Could you check a few things on this model? Use its own coordinates, in mm. A direction names the side the tool comes from. Give positions to 0.01 mm unless a question says otherwise; leave off trailing zeros. Write each loop counter-clockwise with the first axis right and the second up, starting at its lowest first coordinate (ties: lowest second). Pieces come first, ordered by that corner, then holes. Notation, with made-up numbers: (17.25, 28.25) - (42.25, 28.25) arc R24 ccw to (42.25, 65.25) - close; hole circle Ø5 at (89.25, 36). An arc over 180 degrees is marked (long way). Use one line per item in the form item = value.
Autodesk Inventor part; units mm, degrees
ref_plane "YZ Plane" through (0, 0, 0) normal (1, 0, 0) x (0, 1, 0)
ref_plane "XZ Plane" through (0, 0, 0) normal (0, 1, 0) x (-1, 0, 0)
ref_plane "XY Plane" through (0, 0, 0) normal (0, 0, 1) x (1, 0, 0)
sketch "Sketch1" plane through (0, 0, 0) normal (0, 0, 1) x (1, 0, 0)
  circle A0 centre (0, 0) radius 38.1
  dimension "d0" = 76.2
extrude "Extrusion1" add sketch "Sketch1" along normal blind 25.4
fillet "Fillet1" radius 6.35 2 edges at (-38.1, 0, 25.4) (-38.1, 0, 0)
sketch "Sketch3" plane through (0, 0, 25.4) normal (0, 0, 1) x (1, 0, 0)
  line L0 (6.35, 44.45) -> (-53.2838, 44.45)
  circle A0 centre (0, 0) radius 38.1
  arc A1 (-4.3231, -4.6511) -> (6.35, 0) centre (0, 0) ccw
  line L1 (6.35, 0) -> (6.35, 44.45)
  arc A2 (-53.2838, 44.45) -> (-47.6982, 35.6648) centre (-39.6513, 46.9493) ccw
  line L2 (-50.3182, 38.1) -> (-4.3231, -4.6511)
  dimension "d8" = 44.45
  dimension "d9" = 76.2
  dimension "d10" = 12.7
extrude "Extrusion2" add sketch "Sketch3" along normal blind 3.175 contours L1 A0 L2 A2 L0 | L1 A1 L2 A0 picked at (-4.398, 10.0922)
pattern_linear "Rectangular Pattern1" count 2 spacing 28.575 along (0, 0, -1) of "Extrusion2"
sketch "Sketch4" plane through (-53.2838, 44.45, 25.4) normal (0, 1, 0) x (1, 0, 0)
  line L0 (59.6338, -3.175) -> (0, -3.175)
  line L1 (59.6338, 28.575) -> (0, 28.575)
  line L2 (0, -3.175) -> (59.6338, -3.175)
  line L3 (59.6338, -3.175) -> (59.6338, 28.575)
  line L4 (59.6338, 28.575) -> (0, 28.575)
  line L5 (0, 28.575) -> (0, -3.175)
  point P0 (53.2838, 25.4)
  dimension "d20" = 31.75
extrude "Extrusion3" add sketch "Sketch4" along normal blind 3.175
sketch "Sketch5" plane through (-53.2838, 47.625, 25.4) normal (0, 1, 0) x (1, 0, 0)
  circle A0 centre (19.7076, 12.7) radius 25.4
  line L0 (59.6338, 28.575) -> (0, 28.575)
  line L1 (59.6338, -3.175) -> (59.6338, 28.575)
  dimension "d19" = 15.875
  dimension "d21" = 50.8
extrude "Extrusion4" add sketch "Sketch5" along normal blind 3.175
equation "\"d19\" = 0.5 * d20"
properties part number "Caster Placeholder" material "Aluminum 6061"
1. Imagine slicing it at B-B, the plane z = 12.7. List the corners of the cut face in (x, y) for me (3 decimals).
Response values:
outline = (-58.976, 47.625) - (-53.284, 47.625) - (-53.284, 44.45) - (6.35, 44.45) - (6.35, 47.625) - (-8.176, 47.625) - (-8.176, 50.8) - (-58.976, 50.8) - close; circle Ø76.2 at (0, 0)
2. If we mould it in two halves opening along Z, with no side actions, what happens to faces 1 (the face through (-24, 44.45, 13)), 2 (the face through (6.35, 31, 26)), 3 (the face through (7, -7, 0))? For each: pulls with the +Z half, pulls with the -Z half, needs draft (parallel to the pull), parting line crosses it, or undercut.
Response values:
face_1 = undercut
face_2 = needs draft
face_3 = pulls with the -Z half
3. If I drill on line 1 (Z direction, x = -21, y = -8); line 2 (Z direction, x = -37, y = 47.5) (3 decimals); line 3 (Y direction, x = -41, z = 29) (3 decimals), over which ranges is the centre line in solid material (lowest first)? Write a range as from..to.
Response values:
line_1 = 0..25.4
line_2 = -3.175..28.575
line_3 = 47.625..50.8
4. Imagine slicing it at C-C, the plane z = 20.5. List the corners of the cut face in (x, y) for me (3 decimals).
Response values:
outline = (-57.749, 47.625) - (-53.284, 47.625) - (-53.284, 44.45) - (6.35, 44.45) - (6.35, 47.625) - (-9.403, 47.625) - (-9.403, 50.8) - (-57.749, 50.8) - close; circle Ø75.864 at (0, 0)
5. For pin 1 (8.5 mm diameter, centred on x = -14, y = 26.5, fed in from +Z) (3 decimals); pin 2 (12 mm diameter, centred on x = -45.5, y = 29.5, fed in from -Z) (3 decimals); pin 3 (22.5 mm diameter, centred on x = -37, z = 24.5, fed in from -Y), each with a flat end and sliding along its axis, tell me the tip position at first contact or that it passes through.
Response values:
pin_1 = 28.575
pin_2 = -3.175
pin_3 = -27.16
6. Imagine slicing it at A-A, the plane x = 0. List the corners of the cut face in (y, z) for me (3 decimals), and give its area (3 significant figures).
Response values:
outline = (-38.1, 6.35) arc R6.35 ccw to (-31.75, 0) - (-6.35, 0) - (-6.35, -3.175) - (47.625, -3.175) - (47.625, 28.575) - (-6.35, 28.575) - (-6.35, 25.4) - (-31.75, 25.4) arc R6.35 ccw to (-38.1, 19.05) - close; hole (31.75, 0) - (44.45, 0) - (44.45, 25.4) - (31.75, 25.4) arc R6.35 cw to (38.1, 19.05) - (38.1, 6.35) arc R6.35 cw to start
area = 2,320 mm²
7. Which directions (+Z, -Z, +X, -X, +Y, -Y) give clear straight access to the entire face, cutting with the end or side of a thin tool? Please do faces 4 (the face through (-27.64, 17.02, 26.97)), 5 (the face through (-30.235, 23.183, 12.611)), 6 (the face through (-53.284, 46, 12)), 7 (the face through (2.63, -5.78, -1.61)).
Response values:
face_4 = +Z, -X, -Y
face_5 = none
face_6 = +Z, -Z, -X, -Y
face_7 = -Z, -Y
